Verification items for the finished model (mm, model axes). A direction names the side the tool comes from. Coordinates: 2 decimals unless noted, no trailing zeros. Order: outer loops, then holes, each group sorted by start corner. A loop starts at its lowest first (then second) coordinate and runs counter-clockwise, first axis right, second up. Notation, with made-up numbers: (47, 18) -> (65, 18) arc R19 cw to (65, 22) -> close; hole circle Ø10 at (32.25, 2). An arc over 180 degrees is marked (long way). Answer as CSV lines item,"result".
```python
from build123d import *

# Parameters (mm, degrees)
F1_DEPTH = 25.4
F0_W     = 8
F0_H     = 8.7
F2_DEPTH = 2.032
F4_D     = 4.7625


with BuildPart() as f1:
    # F0 (on Front) → F1 (new body)
    with BuildSketch(Plane.XZ):
        Polygon((0, 21.082), (0, 0), (2.032, 0), (2.032, 19.05), (21.1582, 19.05), (21.1582, 0), (23.1902, 0), (23.1902, 21.082), (17.6271, 21.082), (11.5951, 21.082), (5.5631, 21.082), align=None)
        with BuildLine():
            ThreePointArc((15.5951, 25.082), (14.423527, 22.253573), (11.5951, 21.082))
            Line((11.5951, 21.082), (17.6271, 21.082))
            Line((17.6271, 21.082), (17.6271, 33.782))
            Line((17.6271, 33.782), (15.5951, 33.782))
            Line((15.5951, 33.782), (15.5951, 25.082))
        make_face()
        with BuildLine():
            Line((5.5631, 33.782), (5.5631, 21.082))
            Line((5.5631, 21.082), (11.5951, 21.082))
            ThreePointArc((11.5951, 21.082), (8.766673, 22.253573), (7.5951, 25.082))
            Line((7.5951, 25.082), (7.5951, 33.782))
            Line((7.5951, 33.782), (5.5631, 33.782))
        make_face()
    extrude(amount=F1_DEPTH)

    # F0 (on Front) → F2 (join)
    with BuildSketch(Plane.XZ):
        with BuildLine():
            ThreePointArc((7.5951, 25.082), (8.766673, 22.253573), (11.5951, 21.082))
            ThreePointArc((11.5951, 21.082), (14.423527, 22.253573), (15.5951, 25.082))
            Line((15.5951, 25.082), (7.5951, 25.082))
        make_face()
        with Locations((11.5951, 29.432)):
            Rectangle(F0_W, F0_H)
    extrude(amount=F2_DEPTH)

    # F4 (through all)
    with Locations(Plane.YZ.offset(23.1902)):
        with Locations((-12.7, 10.541)):
            Hole(F4_D / 2)


solid = f1.part
```
Item 1: Section check C-C, the plane z = 30.5. Record the boundary of the cut face in (x, y).
Answer list:
outline,"(5.56, -25.4) -> (7.6, -25.4) -> (7.6, -2.03) -> (15.6, -2.03) -> (15.6, -25.4) -> (17.63, -25.4) -> (17.63, 0) -> (5.56, 0) -> close"
Item 2: Section check B-B, the plane y = -12.7. Record the boundary of the cut face in (x, z).
Answer list:
outline,"(0, 0) -> (2.03, 0) -> (2.03, 8.16) -> (0, 8.16) -> close; (0, 12.92) -> (2.03, 12.92) -> (2.03, 19.05) -> (21.16, 19.05) -> (21.16, 12.92) -> (23.19, 12.92) -> (23.19, 21.08) -> (17.63, 21.08) -> (17.63, 33.78) -> (15.6, 33.78) -> (15.6, 25.08) arc R4 cw to (7.6, 25.08) -> (7.6, 33.78) -> (5.56, 33.78) -> (5.56, 21.08) -> (0, 21.08) -> close; (21.16, 0) -> (23.19, 0) -> (23.19, 8.16) -> (21.16, 8.16) -> close"
Item 3: Section check D-D, the plane y = -19.25. Record the boundary of the cut face in (x, z).
Answer list:
outline,"(0, 0) -> (2.03, 0) -> (2.03, 19.05) -> (21.16, 19.05) -> (21.16, 0) -> (23.19, 0) -> (23.19, 21.08) -> (17.63, 21.08) -> (17.63, 33.78) -> (15.6, 33.78) -> (15.6, 25.08) arc R4 cw to (7.6, 25.08) -> (7.6, 33.78) -> (5.56, 33.78) -> (5.56, 21.08) -> (0, 21.08) -> close"
Item 4: Thickness scan on line 1 (X direction, y = -13, z = 5.5); line 2 (X direction, y = -22.5, z = 32); line 3 (Z direction, x = 21.9, y = -12.7). Record the ranges inside material, lowest first.
Answer list:
line 1,"0 to 2.03, 21.16 to 23.19"
line 2,"5.56 to 7.6, 15.6 to 17.63"
line 3,"0 to 8.16, 12.92 to 21.08"
Item 5: Depth check by flat-ended pin: pin 1 Ø1.7 at (x, y) = (1.5, -17) entering from +Z; pin 2 Ø8 at (y, z) = (-6, 14.5) entering from -X; pin 3 Ø9.5 at (y, z) = (-19.5, 30.5) entering from -X; pin 4 Ø2.5 at (y, z) = (-10, 27.5) entering from +X. Enter the tip coordinate at first touch or a pass-through.
Answer list:
pin 1,"z = 21.08"
pin 2,"x = 0"
pin 3,"x = 5.56"
pin 4,"x = 17.63"
Item 6: Tool access check on faces 5 (the flat face through (2.032, -13, 7)), 6 (the flat face through (12, -2.032, 28)), 7 (the flat face through (3, -13, 21.082)), 8 (the flat face through (20, -13, 21.082)). Record the directions out of +Z, -Z, +X, -X, +Y, -Y that give a thin tool (end or side, any length) a straight path to the whole face; none if there is none.
Answer list:
face 5,"-Z, +Y, -Y"
face 6,"+Z, -Y"
face 7,"+Z, -X, +Y, -Y"
face 8,"+Z, +X, +Y, -Y"
Item 7: Release check for a two-part mould opening along X. For faces 1 (the flat face through (11, -13, 19.05)), 2 (the flat face through (17.627, -13, 27)), 3 (the flat face through (0, -15.3, 10.7)), 4 (the flat face through (7, -10, 33.782)) record: +X half, -X half, draft (parallel to the pull), parting line (faces both ways), or undercut.
Answer list:
face 1,"undercut"
face 2,"+X half"
face 3,"-X half"
face 4,"draft"
Item 8: Section check A-A, the plane z = 18. Record the boundary of the cut face in (x, y).
Answer list:
outline,"(0, -25.4) -> (2.03, -25.4) -> (2.03, 0) -> (0, 0) -> close; (21.16, -25.4) -> (23.19, -25.4) -> (23.19, 0) -> (21.16, 0) -> close"
